Source: three-view drawing plus pictorial views. Frame: mm from the lowest corner of the part. A direction names the side the tool comes from. Give positions to 0.01 mm unless a question says otherwise; leave off trailing zeros. Loops run counter-clockwise (first coordinate to the right, second up) from the corner with the lowest first, then second, coordinate; pieces in that order, holes last. Notation, with made-up numbers: (-0.5, 61) -> (39.5, 61) arc R26 ccw to (39.5, 81) -> close; hole circle Ø4 at (2.5, 86.25). An arc over 180 degrees is marked (long way). Answer in a Markdown table with one row per item. Add a question column.
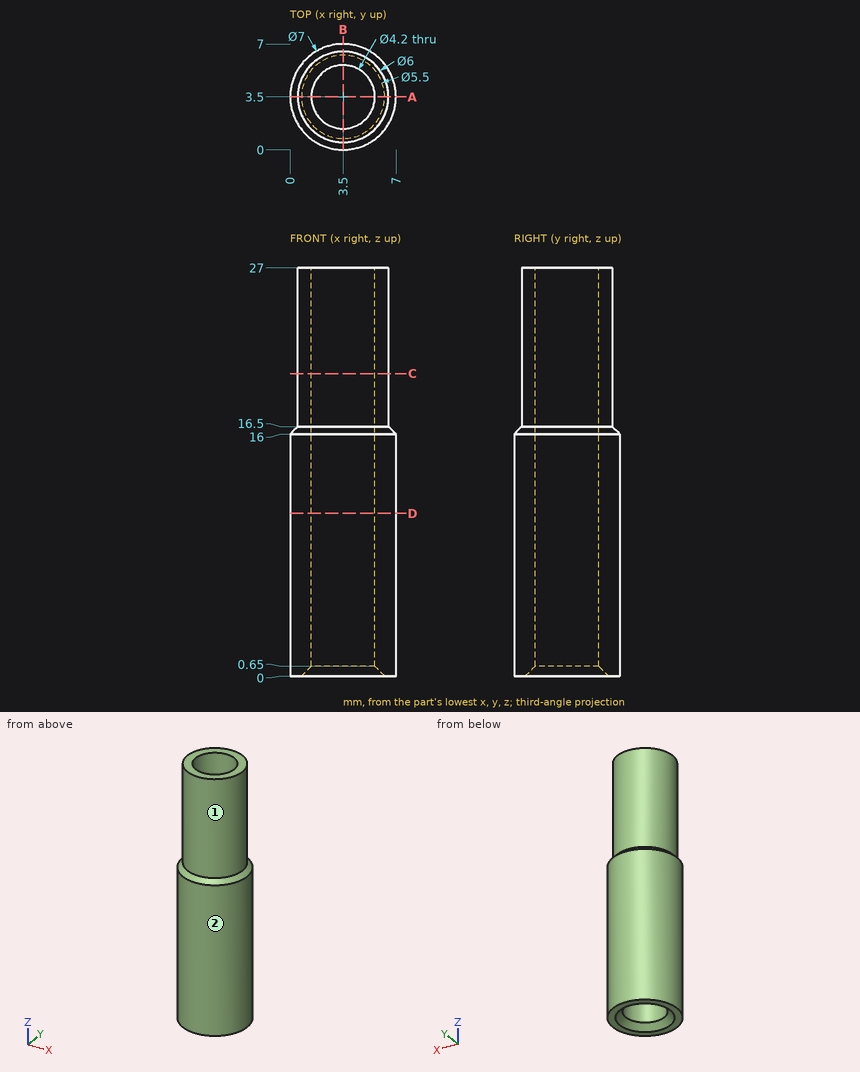
(1) Cut plane D-D on z = 10.75. Return the cut outline in (x, y), then the cut area to 3 significant figures.
(2) Reachability of the marked faces 1 and 2 from +Z, -Z, +X, -X, +Y, -Y: full face, straight path, thin tool, end or side. Return the list, or none.
(3) Pin query (flat end, axial travel): pin 1 Ø4 at (y, z) = (5, 6.5) entering from +X; pin 2 Ø1 at (x, z) = (1, 20) entering from +Y; pin 3 Ø1 at (x, y) = (4, 5.5) entering from -Z; pin 4 Ø1.5 at (y, z) = (6, 10.5) entering from +X. Return the tip coordinate at first contact, or that it passes through.
(4) Cut plane A-A on y = 3.5. Return the cut outline in (x, z), then the cut area to 3 significant figures.
(5) Cut plane C-C on z = 20. Return the cut outline in (x, y), then the cut area to 3 significant figures.
(6) Material intervals for line 1 along Y through (x, z) = (3.5, 6.75); line 2 along X through (y, z) = (2.5, 4.5); line 3 along X through (y, z) = (2.75, 11), sorted ascending. Write a range as from..to.
Answer list:
| question | item | result |
|---|---|---|
| 1 | outline | circle Ø7 at (3.5, 3.5); hole circle Ø4.2 at (3.5, 3.5) |
| 1 | area | 24.6 mm² |
| 2 | face 1 | +Z |
| 2 | face 2 | +Z, -Z |
| 3 | pin 1 | stops at x = 7 |
| 3 | pin 2 | stops at y = 5.74 |
| 3 | pin 3 | stops at z = 0.19 |
| 3 | pin 4 | stops at x = 6.53 |
| 4 | outline | (0, 0) -> (0.75, 0) -> (1.4, 0.65) -> (1.4, 27) -> (0.5, 27) -> (0.5, 16.5) -> (0, 16) -> close; (5.6, 0.65) -> (6.25, 0) -> (7, 0) -> (7, 16) -> (6.5, 16.5) -> (6.5, 27) -> (5.6, 27) -> close |
| 4 | area | 64.4 mm² |
| 5 | outline | circle Ø6 at (3.5, 3.5); hole circle Ø4.2 at (3.5, 3.5) |
| 5 | area | 14.4 mm² |
| 6 | line 1 | y = 0..1.4, 5.6..7 |
| 6 | line 2 | x = 0.15..1.65, 5.35..6.85 |
| 6 | line 3 | x = 0.08..1.54, 5.46..6.92 |
